The model under review builds one solid part; all positions refer to its coordinate system, in mm. Coordinates: 2 decimals unless noted, no trailing zeros. One line per question, with ' | ' between items. Start each with the question number.
from build123d import *

# Parameters (mm, degrees)
ESQUISSE1_W             = 203.2
ESQUISSE1_H             = 76.2
BOSS_EXTRU_1_DEPTH      = 12.7
ESQUISSE2_R             = 1.666875
ENL_V_MAT_EXTRU_1_DEPTH = 110.249530891


with BuildPart() as part:
    # Esquisse1 → Boss.-Extru.1 (new body)
    with BuildSketch(Plane.XY):
        Rectangle(ESQUISSE1_W, ESQUISSE1_H)
    extrude(amount=BOSS_EXTRU_1_DEPTH)

    # Esquisse2 → Enlèv. mat.-Extru.1 (cut, through all)
    with BuildSketch(Plane(origin=(0, 0, 0), x_dir=(-1, 0, 0), z_dir=(0, 0, -1))):
        with Locations((81.49209, 0)):
            Circle(ESQUISSE2_R)
        with Locations((66.67627, 0)):
            Circle(ESQUISSE2_R)
        with Locations((51.86045, 0)):
            Circle(ESQUISSE2_R)
        with Locations((37.04463, 0)):
            Circle(ESQUISSE2_R)
        with Locations((22.22881, 0)):
            Circle(ESQUISSE2_R)
        with Locations((7.41299, 0)):
            Circle(ESQUISSE2_R)
        with Locations((-7.40283, 0)):
            Circle(ESQUISSE2_R)
        with Locations((-22.21865, 0)):
            Circle(ESQUISSE2_R)
        with Locations((-37.03447, 0)):
            Circle(ESQUISSE2_R)
        with Locations((-51.85029, 0)):
            Circle(ESQUISSE2_R)
        with Locations((-66.66611, 0)):
            Circle(ESQUISSE2_R)
        with Locations((-81.48193, 0)):
            Circle(ESQUISSE2_R)
    extrude(amount=-ENL_V_MAT_EXTRU_1_DEPTH, mode=Mode.SUBTRACT)


solid = part.part
1) Wall thickness on L1, parallel to Y at x = 65.5, z = 1.5; L2, parallel to Y at x = -38, z = 3.5: over which ranges is each line inside the solid? List them lowest first.
2) Mouldability with a two-part tool opening along Y and no side actions: class faces 1 (the face through (-20.564, 0.073, 6.261)), 2 (the face through (-9.003, 0.501, 6.261)), 3 (the face through (-101.6, -1, 6)), 4 (the face through (-1, 38.1, 6)) as +Y half, -Y half, draft (parallel to the pull), parting line (faces both ways), or undercut.
3) Insertion check: pin 1 Ø4 at (x, y) = (81.48, 0) entering from +Z. The pin has a flat end and moves straight along its axis. Give the tip position at first contact, or say it passes through.
Filled sheet:
1) L1: -38.1 to -1.19, 1.19 to 38.1 | L2: -38.1 to -1.37, 1.37 to 38.1
2) face 1: undercut | face 2: undercut | face 3: draft | face 4: +Y half
3) pin 1: z = 12.7
